Verification items for this drawing (mm, ordinates from the low corner). Coordinates: 2 decimals unless noted, no trailing zeros. Write each loop counter-clockwise with the first axis right and the second up, starting at its lowest first coordinate (ties: lowest second). Pieces come first, ordered by that corner, then holes. Notation, with made-up numbers: (82, 79.25) -> (114, 79.25) arc R30 cw to (114, 114.25) -> close; hole circle Ø9 at (7, 27). An arc over 180 degrees is marked (long way). Put each result on its own line as item: value. Start each with the question number.
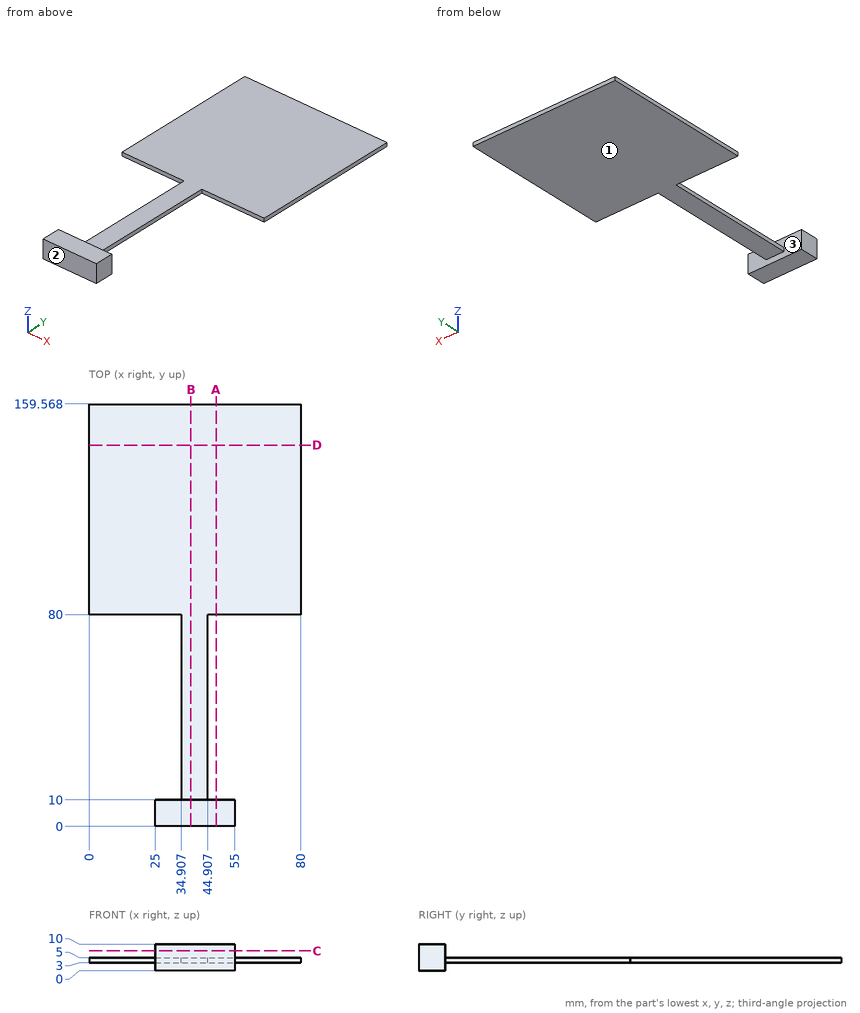
Item 1: Go/stop test with flat-tipped pins: P1, Ø1, axis at y = 33.5, z = 3.5, coming from the -X side; P2, Ø0.6, axis at x = 13.5, z = 3.5, coming from the -Y side; P3, Ø0.6, axis at y = 61.5, z = 4, coming from the +X side. Record where each tip stops, or that it passes through.
Item 2: Section check A-A, the plane x = 48. Enter the section's corners in (y, z), and give its area (3 significant figures).
Item 3: Section check D-D, the plane y = 144. Enter the section's corners in (x, z), and give its area (3 significant figures).
Item 4: Scan lines: line 1 along Y through (x, z) = (52.5, 7.5); line 2 along Z through (x, y) = (33, 81); line 3 along Y through (x, z) = (49, 4.75). Record each from-to range of solid material in increasing order. Write a range as [from, to].
Item 5: Section check C-C, the plane z = 7.5. Enter the section's corners in (x, y), and give its area (3 significant figures).
Item 6: Mould release check, pull along Y, two halves, no side actions. Record for the marked faces 1, 2 and 3: released by +Y, released by -Y, zero draft, split by the parting line, or undercut.
Item 7: Section check B-B, the plane x = 38.5. Enter the section's corners in (y, z).
From the geometry:
1. P1: x = 34.91
1. P2: y = 80
1. P3: x = 44.91
2. outline: (0, 0) -> (10, 0) -> (10, 10) -> (0, 10) -> close; (80, 3) -> (159.57, 3) -> (159.57, 5) -> (80, 5) -> close
2. area: 259 mm²
3. outline: (0, 3) -> (80, 3) -> (80, 5) -> (0, 5) -> close
3. area: 160 mm²
4. line 1: [0, 10]
4. line 2: [3, 5]
4. line 3: [0, 10], [80, 159.57]
5. outline: (25, 0) -> (55, 0) -> (55, 10) -> (25, 10) -> close
5. area: 300 mm²
6. face 1: zero draft
6. face 2: released by -Y
6. face 3: undercut
7. outline: (0, 0) -> (10, 0) -> (10, 3) -> (159.57, 3) -> (159.57, 5) -> (10, 5) -> (10, 10) -> (0, 10) -> close
